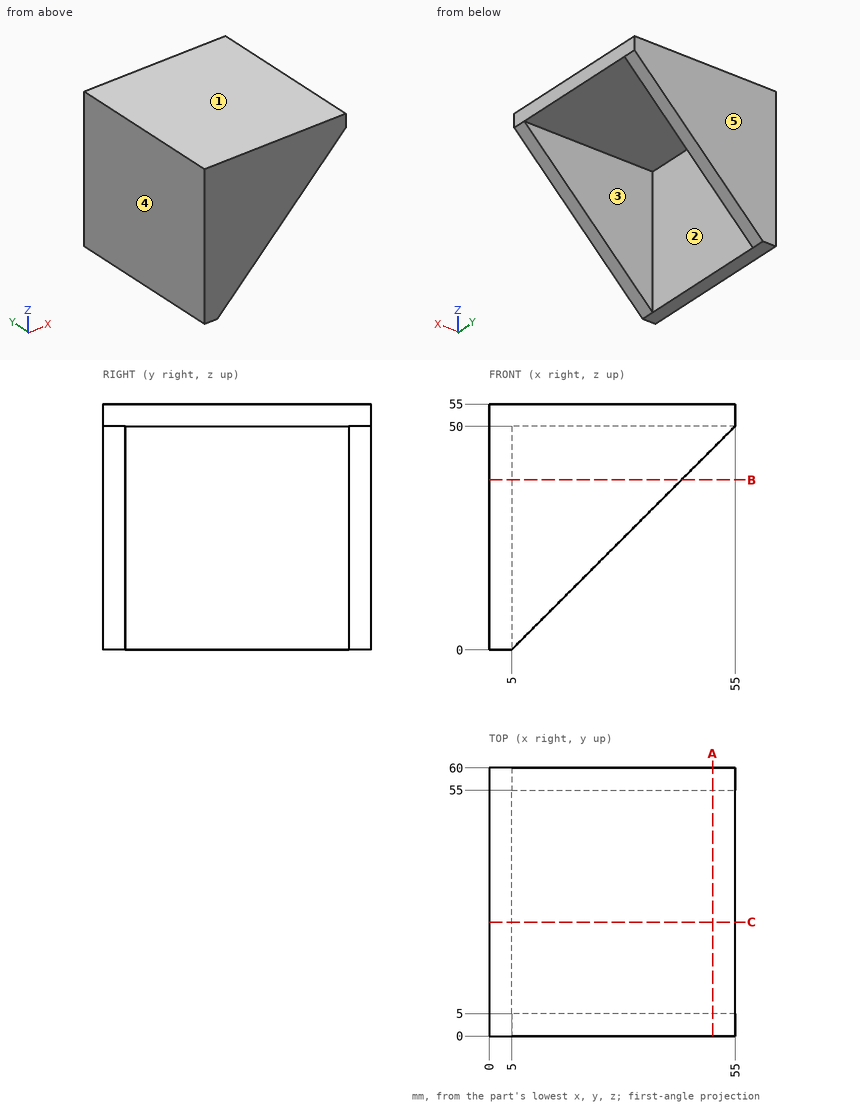
Verification items for this drawing (mm, ordinates from the low corner). A direction names the side the tool comes from. Coordinates: 2 decimals unless noted, no trailing zeros. Write each loop counter-clockwise with the first axis right and the second up, starting at its lowest first coordinate (ties: lowest second). Pieces come first, ordered by that corner, then holes. Notation, with made-up numbers: (-28.5, -23.5) -> (4.5, -23.5) arc R27 cw to (4.5, 13.5) -> close; hole circle Ø5 at (-23.5, -16.5). An arc over 180 degrees is marked (long way). One line per item, written item: value. Start each with the question number.
Q1. Mould release check, pull along Y, two halves, no side actions. Record for the marked faces 3, 4 and 5: pulls with the +Y half, pulls with the -Y half, needs draft (parallel to the pull), parting line crosses it, or undercut.
Q2. Cross-section at C-C on y = 25.5. Enter the section's corners in (x, z), and give its area (3 significant figures).
Q3. Go/stop test with flat-tipped pins: P1, Ø4, axis at y = 8, z = 24.5, coming from the +X side; P2, Ø12, axis at y = 37.5, z = 43.5, coming from the -X side; P3, Ø4, axis at x = 38.5, y = 18, coming from the -Z side. Record where each tip stops, or that it passes through.
Q4. Access from +Z, -Z, +X, -X, +Y, -Y to the whole of each face (thin tool, end or side, straight path). Record for the marked faces 1 and 2.
Q5. Cross-section at B-B on z = 38. Enter the section's corners in (x, y).
Q6. Thickness scan on L1, parallel to Y at x = 23, z = 29; L2, parallel to Z at x = 23, y = 11; L3, parallel to X at y = 27.5, z = 19.5. Record the ranges inside material, lowest first. Write a range as from..to.
Q7. Cross-section at A-A on x = 50. Enter the section's corners in (y, z).
Checked values:
1. face 3: undercut
1. face 4: needs draft
1. face 5: pulls with the +Y half
2. outline: (0, 0) -> (5, 0) -> (5, 50) -> (55, 50) -> (55, 55) -> (0, 55) -> close
2. area: 525 mm²
3. P1: stops at x = 5
3. P2: stops at x = 0
3. P3: stops at z = 50
4. face 1: +Z, +X, -X, +Y, -Y
4. face 2: -Z, +X
5. outline: (0, 0) -> (43, 0) -> (43, 5) -> (5, 5) -> (5, 55) -> (43, 55) -> (43, 60) -> (0, 60) -> close
6. L1: y = 0..5, 55..60
6. L2: z = 50..55
6. L3: x = 0..5
7. outline: (0, 45) -> (5, 45) -> (5, 50) -> (55, 50) -> (55, 45) -> (60, 45) -> (60, 55) -> (0, 55) -> close
